```python
from build123d import *

# Parameters (mm, degrees)
F0_R     = 6
F1_DEPTH = 2
F2_SIZE2 = 2.5980762114
F2_SIZE  = 1.5
F4_R     = 2.25
F4_R_2   = 1.4
F5_DEPTH = 7
F6_R     = 1.2


# Not quite as in the source:
# - a fillet or chamfer that OpenCascade refuses, or shapes differently, is made with other operations: its cross-section is extruded or revolved along the edge and cut away or added


with BuildPart() as f1:
    # F0 (on Top) → F1 (new body)
    with BuildSketch(Plane.XY):
        Circle(F0_R)
    extrude(amount=F1_DEPTH)

    # F2
    f2_edges = [f1.edges().sort_by_distance(p)[0] for p in [
        (-6, 0, 0),
    ]]
    f2_side = f1.faces().sort_by_distance((-6, 0, 1))[0]
    chamfer(f2_edges, length=F2_SIZE, length2=F2_SIZE2, reference=f2_side)

    # F3: fillet of radius 1 on 2 edges, made by hand

    # F3_s1 → F3_t2 (revolve, cut)
    with BuildSketch(Plane.XZ):
        with BuildLine():
            ThreePointArc((3.6339745962, 0.1339745962), (3.3927936413, 0.0340741737), (3.1339745962, 0))
            Line((3.1339745962, 0), (3.4019237886, 0))
            Line((3.4019237886, 0), (3.6339745962, 0.1339745962))
        make_face()
    revolve(axis=Axis((0, 0, 0), (0, 0, 1)), mode=Mode.SUBTRACT)

    # F3_s3 → F3_t4 (revolve, cut)
    with BuildSketch(Plane.XZ):
        with BuildLine():
            ThreePointArc((6, 2), (5.8486778537, 1.5452494356), (5.5031382462, 1.2131367327))
            Line((5.5031382462, 1.2131367327), (6, 1.5))
            Line((6, 1.5), (6, 2))
        make_face()
    revolve(axis=Axis((0, 0, 1.5), (0, 0, 1)), mode=Mode.SUBTRACT)

    # F4 (on face) → F5 (join)
    with BuildSketch(Plane.XY.offset(2)):
        Circle(F4_R)
        Circle(F4_R_2, mode=Mode.SUBTRACT)
    extrude(amount=F5_DEPTH)

    # F6
    f6_edges = [f1.edges().sort_by_distance(p)[0] for p in [
        (-1.4, 0, 2),
    ]]
    fillet(f6_edges, radius=F6_R)


solid = f1.part
```
Read the model definition and answer for the solid it produces. Units are mm, in the model's axes. Coordinates: 2 decimals unless noted, no trailing zeros. Write each loop counter-clockwise with the first axis right and the second up, starting at its lowest first coordinate (ties: lowest second). Pieces come first, ordered by that corner, then holes. Notation, with made-up numbers: (40.5, -23.75) - (51.5, -23.75) arc R30 ccw to (51.5, 6.25) - close; hole circle Ø2 at (42.25, 10.25). An arc over 180 degrees is marked (long way). Answer as a JSON object with one key per item and string values. Group by question number.
1. The mould has two halves that part along Y. Classify faces 1 (the cylindrical face through (-0.29, 2.23, 5.45)), 2 (the flat face through (3, 0, 2)), 3 (the cylindrical face through (-1.4, 0.06, 6.06)): +Y half, -Y half, draft (parallel to the pull), parting line (faces both ways), or undercut.
2. A cutting plane is placed at A-A (z = 5.75). Determine the outline of the cut face in (x, y).
3. Each of these flat-tipped pins is pushed along its axis until it touches: P1, Ø1, axis at y = 1.5, z = 8, coming from the -X side; P2, Ø2, axis at x = 3, z = 7, coming from the -Y side. Where does it stop, or does it pass through?
4. Consider L1, parallel to Y at x = 0, z = 7.45; L2, parallel to X at y = -0.25, z = 3.5; L3, parallel to Z at x = -3, y = 1. Determine where each line is inside the solid, lowest interval first. Write a range as [from, to].
Worked out:
{
 "1": {"face 1": "parting line", "face 2": "draft", "face 3": "undercut"},
 "2": {"outline": "circle Ø4.5 at (0, 0); hole circle Ø2.8 at (0, 0)"},
 "3": {"P1": "stops at x = -2.02", "P2": "stops at y = -1.03"},
 "4": {"L1": "y = [-2.25, -1.4], [1.4, 2.25]", "L2": "x = [-2.24, -1.38], [1.38, 2.24]", "L3": "z = [0, 2]"}
}
